from build123d import *

# Parameters (mm, degrees)
F1_DEPTH = 15
F2_R     = 7.5
F3_DEPTH = 200.658232
F4_R     = 10
F5_DEPTH = 70


with BuildPart() as f1:
    # F0 (on Front) → F1 (new body, symmetric)
    with BuildSketch(Plane.XZ):
        with BuildLine():
            ThreePointArc((-21.213203, 21.213203), (0, 30), (21.213203, 21.213203))
            Line((21.213203, 21.213203), (70.710678, 70.710678))
            ThreePointArc((70.710678, 70.710678), (0, 100), (-70.710678, 70.710678))
            Line((-70.710678, 70.710678), (-21.213203, 21.213203))
        make_face()
    extrude(amount=F1_DEPTH, both=True)

    # F2 (on Top) → F3 (cut)
    with BuildSketch(Plane.XY):
        Circle(F2_R)
    extrude(amount=F3_DEPTH, mode=Mode.SUBTRACT)

    # F4 (on Top) → F5 (cut)
    with BuildSketch(Plane.XY):
        Circle(F4_R)
    extrude(amount=F5_DEPTH, mode=Mode.SUBTRACT)


solid = f1.part
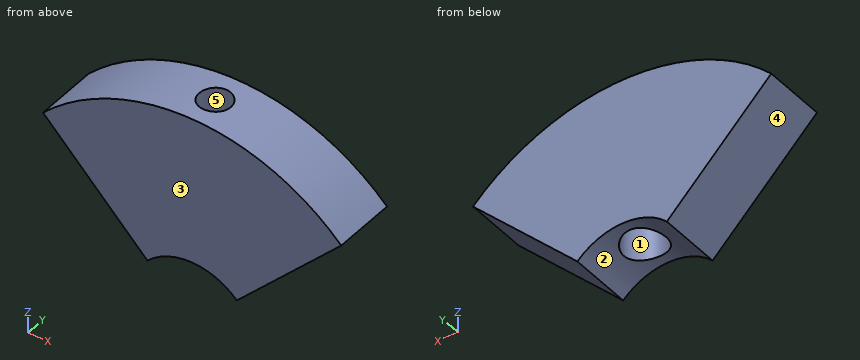
CAD build for the part. Positions are in the model's coordinates, mm. Face numbers are marked on the shaded views. A direction names the side the tool comes from. Coordinates: 2 decimals unless noted, no trailing zeros. Order: outer loops, then holes, each group sorted by start corner. A loop starts at its lowest first (then second) coordinate and runs counter-clockwise, first axis right, second up. Notation, with made-up numbers: (-27.5, 55) -> (27.5, 55) arc R16 cw to (27.5, 63) -> close; hole circle Ø7 at (-26.5, 4.5). An arc over 180 degrees is marked (long way). Answer in a Markdown table with one row per item.
1) Drill centre lines: line 1 (Y direction, x = 0, z = 53.5); line 2 (Z direction, x = 2.5, y = -8.5); line 3 (X direction, y = 0, z = 88). Where is each one in solid material? Low to high.
Check values:
| item | result |
|---|---|
| line 1 | -15 to -10, 10 to 15 |
| line 2 | 70 to 99.97 |
| line 3 | -47.5 to -7.5, 7.5 to 47.5 |
2) Flat gauge pins, fed straight in: P1, Ø10, axis at x = 1, y = 4.5, coming from the -Z side; P2, Ø2, axis at y = -7.5, z = 66.5, coming from the +X side; P3, Ø12, axis at x = -16, y = -10.5, coming from the +Z side. Where does each tip first touch, or does it go through?
Check values:
| item | result |
|---|---|
| P1 | z = 70 |
| P2 | x = 67.5 |
| P3 | z = 99.5 |
3) Band-saw the part on B-B (y = 0). List the corners of the cut face in (x, z).
Check values:
| item | result |
|---|---|
| outline | (-70.71, 70.71) -> (-21.21, 21.21) arc R30 cw to (-10, 28.28) -> (-10, 70) -> (-7.5, 70) -> (-7.5, 99.72) arc R100 ccw to start; (7.5, 70) -> (10, 70) -> (10, 28.28) arc R30 cw to (21.21, 21.21) -> (70.71, 70.71) arc R100 ccw to (7.5, 99.72) -> close |
4) Mould opens along X. For the marked faces 3, 4 and 5 say: pulls with the +X half, pulls with the -X half, needs draft (parallel to the pull), parting line crosses it, or undercut.
Check values:
| item | result |
|---|---|
| face 3 | needs draft |
| face 4 | pulls with the -X half |
| face 5 | undercut |
5) Which spindle directions (+Z, -Z, +X, -X, +Y, -Y) get a long thin tool onto all of the face, cutting with end or side? Do the marked faces 1 and 2. Say none if no direction does.
Check values:
| item | result |
|---|---|
| face 1 | -Z |
| face 2 | -Z, +Y, -Y |
6) Band-saw the part on C-C (z = 91). List the corners of the cut face in (x, y).
Check values:
| item | result |
|---|---|
| outline | (-41.46, -15) -> (41.46, -15) -> (41.46, 15) -> (-41.46, 15) -> close; hole circle Ø15 at (0, 0) |
7) Band-saw the part on D-D (y = -12). List the corners of the cut face in (x, z).
Check values:
| item | result |
|---|---|
| outline | (-70.71, 70.71) -> (-21.21, 21.21) arc R30 cw to (21.21, 21.21) -> (70.71, 70.71) arc R100 ccw to start |
8) Band-saw the part on A-A (x = 0). List the corners of the cut face in (y, z), and give its area (3 significant figures).
Check values:
| item | result |
|---|---|
| outline | (-15, 30) -> (-10, 30) -> (-10, 70) -> (-7.5, 70) -> (-7.5, 100) -> (-15, 100) -> close; (7.5, 70) -> (10, 70) -> (10, 30) -> (15, 30) -> (15, 100) -> (7.5, 100) -> close |
| area | 850 mm2 |
